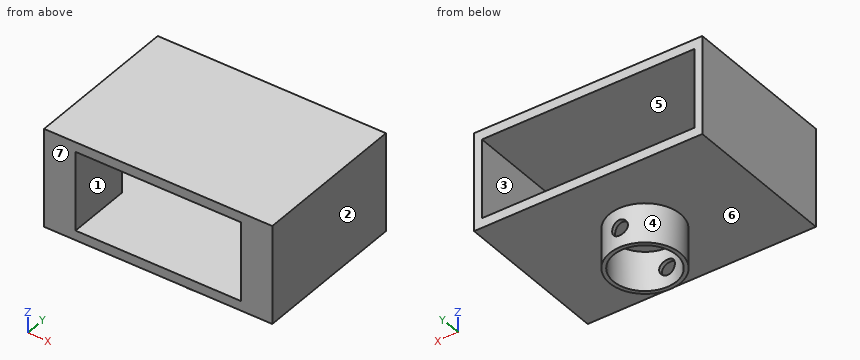
Autodesk Inventor part; units mm, degrees
ref_plane "YZ Plane" through (0, 0, 0) normal (1, 0, 0) x (0, 1, 0)
ref_plane "XZ Plane" through (0, 0, 0) normal (0, 1, 0) x (-1, 0, 0)
ref_plane "XY Plane" through (0, 0, 0) normal (0, 0, 1) x (1, 0, 0)
sketch "Esquisse1" plane through (0, 0, 0) normal (0, 1, 0) x (-1, 0, 0)
  line L0 (0, 0) -> (0, 2.45)
  line L1 (0, 0) -> (2.45, 0) construction
  line L2 (0, 2.45) -> (27, 2.45)
  line L3 (27, 2.45) -> (27, 22.55)
  line L4 (27, 22.55) -> (-27, 22.55)
  line L5 (-27, 22.55) -> (-27, 2.45)
  line L6 (-27, 2.45) -> (0, 2.45)
  line L7 (0, 0) -> (29, 0)
  line L8 (29, 0) -> (29, 25)
  line L9 (29, 25) -> (-29, 25)
  line L10 (-29, 25) -> (-29, 0)
  line L11 (-29, 0) -> (0, 0)
  dimension "d0" = 2.45
  dimension "d1" = 90
  dimension "d2" = 27
  dimension "d3" = 20.1
  dimension "d4" = 54
  dimension "d5" = 29
  dimension "d6" = 25
  dimension "d7" = 58
extrude "Extrusion1" add sketch "Esquisse1" along normal blind 40
sketch "Esquisse2" plane through (29, 0, 0) normal (0, 0, -1) x (-1, 0, 0)
  line L0 (29, 0) -> (29, 40)
  line L1 (58, 40) -> (0, 40)
  line L2 (0, 0) -> (0, 40)
  line L3 (0, 20) -> (58, 20)
  line L4 (58, 0) -> (58, 40)
  circle A0 centre (29, 20) radius 8
  circle A1 centre (29, 20) radius 9
  dimension "d10" = 16
  dimension "d11" = 18
extrude "Extrusion2" add sketch "Esquisse2" along normal blind 10 contours A1 L3 A0 L0 | L0 A0 L3 A1 | A1 L0 A0 L3 | L3 A0 L0 A1
sketch "Esquisse3" plane through (0, 0, 0) normal (0, 1, 0) x (-1, 0, 0)
  line L0 (-9, -10) -> (9, -10)
  line L1 (0, -10) -> (0, -5)
  point P0 (0, 0)
  dimension "d14" = 5
hole "Perçage1" at (0, 0, -5) direction (0, 1, 0) diameter 4 end through all
sketch "Esquisse4" plane through (0, 0, 0) normal (0, -1, 0) x (1, 0, 0)
  line L0 (27, 2.45) -> (27, 22.55)
  line L1 (27, 22.55) -> (-27, 22.55)
  line L2 (-27, 2.45) -> (27, 2.45)
  line L3 (-27, 22.55) -> (-27, 2.45)
  line L4 (27, 22.55) -> (21, 22.55)
  line L5 (27, 22.55) -> (33, 22.55) construction
  line L6 (21, 22.55) -> (21, 2.45)
  line L7 (-27, 22.55) -> (-21, 22.55)
  line L8 (-21, 22.55) -> (-21, 2.45)
  point P0 (0, 0)
  dimension "d22" = 6
  dimension "d23" = 180
  dimension "d24" = 6
extrude "Extrusion3" add sketch "Esquisse4" against normal blind 16.4 contours L2 L6 L1 L0 | L2 L3 L1 L8
sketch "Esquisse5" plane through (0, 16.4, 0) normal (0, 1, 0) x (1, 0, 0)
  line L0 (-21, -22.55) -> (-21, -2.45)
  line L1 (-21, -22.55) -> (-21, -12.5)
  line L2 (-21, -12.5) -> (-21, -11.5)
  line L3 (-27, -22.55) -> (-27, -2.45)
  line L4 (-21, -11.5) -> (-27, -11.5)
  line L5 (-21, -12.5) -> (-21, -13.5)
  line L6 (-21, -13.5) -> (-27, -13.5)
  line L7 (0, -14.9752) -> (0, -10.0185)
  line L8 (21, -22.55) -> (21, -2.45)
  line L9 (27, -22.55) -> (27, -2.45)
  line L10 (21, -11.5) -> (27, -11.5)
  line L11 (21, -13.5) -> (27, -13.5)
  point P0 (0, 0)
  dimension "d27" = 10.05
  dimension "d28" = 1
  dimension "d29" = 1
extrude "Extrusion4" cut sketch "Esquisse5" against normal blind 2
sketch "Esquisse6" plane through (0, 16.4, 0) normal (0, 1, 0) x (1, 0, 0)
  line L0 (-27, -22.55) -> (-27, -2.45)
  line L1 (-21, -22.55) -> (-21, -13.5)
  line L2 (-21, -11.5) -> (-21, -2.45)
  line L3 (-27, -12.5) -> (-27, -17.5)
  line L4 (-27, -17.5) -> (-24.775, -17.5)
  line L5 (-24.775, -17.5) -> (-24.775, -7.5)
  line L6 (0, -16.5029) -> (0, -8.8773)
  point P0 (0, 0)
  point P1 (24.775, -17.5)
  point P2 (24.775, -7.5)
  dimension "d32" = 5
  dimension "d33" = 2.225
  dimension "d34" = 10
hole "Perçage2" at (-24.775, 16.4, 17.5) at (-24.775, 16.4, 7.5) at (24.775, 16.4, 17.5) at (24.775, 16.4, 7.5) direction (0, -1, 0) diameter 3.242 depth 11.8 tip angle 118
properties part number "Attache servomoteur_bogie"
Work out the finished part from the listing and answer in its coordinate system (mm). Face numbers are marked on the shaded views. A direction names the side the tool comes from. Coordinates: 2 decimals unless noted, no trailing zeros. Loops run counter-clockwise (first coordinate to the right, second up) from the corner with the lowest first, then second, coordinate; pieces in that order, holes last. Notation, with made-up numbers: M 2,10 L 48,10 A28 cw 48,47 Z; hole C 65.5,71 d4. An arc over 180 degrees is marked long. Answer in a Markdown table with one row per item. Add a question column.
1. Flat-ended cylindrical pins translate along their axes: P1, Ø5, axis at x = -10.5, y = 27, coming from the -Z side; P2, Ø3, axis at x = 22.5, z = 18, coming from the +Y side; P3, Ø5, axis at x = 0, z = -5, coming from the +Y side; P4, Ø2.5, axis at x = 0, z = -5, coming from the -Y side. Find the tip coordinate at first contact, or state that the pin passes through.
2. Find section A-A, the plane x = 0. Write down the section's boundary in (y, z).
3. Consider L1, parallel to X at y = 9, z = 7.5; L2, parallel to X at y = 25.5, z = 6; L3, parallel to Z at x = 22, y = 14.5. Determine where each line is inside the solid, lowest interval first.
4. Find section D-D, the plane x = 16.5. Write down the section's boundary in (y, z), then the cut area to 3 significant figures.
5. Find section B-B, the plane y = 33. Write down the section's boundary in (x, z), then the cut area to 3 significant figures.
6. Find section C-C, the plane z = 4.5. Write down the section's boundary in (x, y), then the cut area to 3 significant figures.
7. The mould has two halves that part along Z. Classify the marked faces 5, 6 and 7: pulls with the +Z half, pulls with the -Z half, needs draft (parallel to the pull), parting line crosses it, or undercut.
8. A tool of negligible diameter and unlimited length cuts with its end or side. For the marked faces 1, 2, 3 and 4, from which of +Z, -Z, +X, -X, +Y, -Y can it reach the whole face along a straight path? Write none if from no direction.
Reported:
| question | item | result |
|---|---|---|
| 1 | P1 | stops at z = 0 |
| 1 | P2 | stops at y = 16.4 |
| 1 | P3 | stops at y = 29 |
| 1 | P4 | passes through |
| 2 | outline | M 0,0 L 11,0 L 11,-3 L 12,-3 L 12,0 L 28,0 L 28,-3 L 29,-3 L 29,0 L 40,0 L 40,2.45 L 0,2.45 Z; M 0,22.55 L 40,22.55 L 40,25 L 0,25 Z; M 11,-10 L 12,-10 L 12,-7 L 11,-7 Z; M 28,-10 L 29,-10 L 29,-7 L 28,-7 Z |
| 3 | L1 | x = -29 to -26.4, -23.15 to -21, 21 to 23.15, 26.4 to 29 |
| 3 | L2 | x = -29 to -27, 27 to 29 |
| 3 | L3 | z = 0 to 11.5, 13.5 to 25 |
| 4 | outline | M 0,0 L 40,0 L 40,2.45 L 0,2.45 Z; M 0,22.55 L 40,22.55 L 40,25 L 0,25 Z |
| 4 | area | 196 mm^2 |
| 5 | outline | M -29,0 L 29,0 L 29,25 L -29,25 Z; hole M -27,2.45 L 27,2.45 L 27,22.55 L -27,22.55 Z |
| 5 | area | 365 mm^2 |
| 6 | outline | M -29,0 L -21,0 L -21,16.4 L -27,16.4 L -27,40 L -29,40 Z; M 21,0 L 29,0 L 29,40 L 27,40 L 27,16.4 L 21,16.4 Z |
| 6 | area | 357 mm^2 |
| 7 | face 5 | undercut |
| 7 | face 6 | pulls with the -Z half |
| 7 | face 7 | needs draft |
| 8 | face 1 | +Y, -Y |
| 8 | face 2 | +Z, -Z, +X, +Y, -Y |
| 8 | face 3 | +Y |
| 8 | face 4 | -Z |
